The listing builds one solid part. Answer for the finished solid, in the listing's coordinates (mm). A direction names the side the tool comes from. Give positions to 0.01 mm unless a question says otherwise; leave off trailing zeros. Write each loop counter-clockwise with the first axis right and the second up, starting at its lowest first coordinate (ties: lowest second). Pieces come first, ordered by that corner, then holes.
```python
from build123d import *

# Parameters (mm, degrees)
SZKIC1_R                      = 8.5
SZKIC1_R_2                    = 4.2
DODANIE_WYCI_GNI_CIE1_DEPTH   = 30
SZKIC1_W                      = 60
SZKIC1_H                      = 5
DODANIE_WYCI_GNI_CIE1_2_DEPTH = 30
DODANIE_WYCI_GNI_CIE2_DEPTH   = 5
SZKIC3_W                      = 6
SZKIC3_H                      = 22
DODANIE_WYCI_GNI_CIE3_DEPTH   = 26
DODANIE_WYCI_GNI_CIE4_DEPTH   = 5
WYTNIJ_WYCI_GNI_CIE1_REACH    = 62.052
SZKIC5_R                      = 2
WYTNIJ_WYCI_GNI_CIE2_REACH    = 62.052
SZKIC6_W                      = 10.270986067
SZKIC6_H                      = 1.5
SZKIC7_W                      = 9.24961725
SZKIC7_H                      = 2.5
DODANIE_WYCI_GNI_CIE5_DEPTH   = 30
SZKIC8_R                      = 2
WYTNIJ_WYCI_GNI_CIE3_DEPTH    = 30


with BuildPart() as part:
    # Szkic1 → Dodanie-wyci_gni_cie1 (new body)
    with BuildSketch(Plane(origin=(0, 0, 0), x_dir=(1, 0, 0), z_dir=(0, 1, 0))):
        with Locations(Location((0, 34, 0), (0, 0, 270))):
            Circle(SZKIC1_R)
        with Locations(Location((0, 34, 0), (0, 0, 270))):
            Circle(SZKIC1_R_2, mode=Mode.SUBTRACT)
    extrude(amount=DODANIE_WYCI_GNI_CIE1_DEPTH)



with BuildPart() as body_2:
    # Szkic1 → Dodanie-wyci_gni_cie1 2 (new body)
    with BuildSketch(Plane(origin=(0, 0, 0), x_dir=(1, 0, 0), z_dir=(0, 1, 0))):
        with Locations((0, 2.5)):
            Rectangle(SZKIC1_W, SZKIC1_H)
    extrude(amount=DODANIE_WYCI_GNI_CIE1_2_DEPTH)


with BuildPart() as part_1:
    add(part.part)

    add(body_2.part)  # Dodanie-wyci_gni_cie2 merges body 2
    # Szkic2 → Dodanie-wyci_gni_cie2 (add)
    with BuildSketch(Plane.XZ):
        Polygon((30, -5), (8.5, -34), (0, -25.5), (-8.5, -34), (-30, -5), align=None)
    extrude(amount=-DODANIE_WYCI_GNI_CIE2_DEPTH)

    # Szkic3 → Dodanie-wyci_gni_cie3 (add)
    with BuildSketch(Plane(origin=(0, 30, 0), x_dir=(1, 0, 0), z_dir=(0, 1, 0))):
        with Locations((0, 16)):
            Rectangle(SZKIC3_W, SZKIC3_H)
    extrude(amount=-DODANIE_WYCI_GNI_CIE3_DEPTH)

    # Szkic4 → Dodanie-wyci_gni_cie4 (add)
    with BuildSketch(Plane(origin=(0, 30, 0), x_dir=(1, 0, 0), z_dir=(0, 1, 0))):
        Polygon((0, 26.824162036), (8.5, 34), (30, 5), (-30, 5), (-8.5, 34), align=None)
    extrude(amount=-DODANIE_WYCI_GNI_CIE4_DEPTH)

    # Szkic5 → Wytnij-wyci_gni_cie1 (cut, up to next)
    with BuildSketch(Plane.XY, mode=Mode.PRIVATE) as wytnij_wyci_gni_cie1_sk1:
        with Locations((-20, 15)):
            Circle(SZKIC5_R)
    wytnij_wyci_gni_cie1_tool1 = extrude(wytnij_wyci_gni_cie1_sk1.sketch, amount=-WYTNIJ_WYCI_GNI_CIE1_REACH, mode=Mode.PRIVATE) & part_1.part
    # Szkic5 → Wytnij-wyci_gni_cie1 (cut, up to next)
    with BuildSketch(Plane.XY, mode=Mode.PRIVATE) as wytnij_wyci_gni_cie1_sk2:
        with Locations((20, 15)):
            Circle(SZKIC5_R)
    wytnij_wyci_gni_cie1_tool2 = extrude(wytnij_wyci_gni_cie1_sk2.sketch, amount=-WYTNIJ_WYCI_GNI_CIE1_REACH, mode=Mode.PRIVATE) & part_1.part
    add(wytnij_wyci_gni_cie1_tool1.solids().sort_by_distance((-20, 15, 0))[0], mode=Mode.SUBTRACT)
    add(wytnij_wyci_gni_cie1_tool2.solids().sort_by_distance((20, 15, 0))[0], mode=Mode.SUBTRACT)

    # Szkic6 → Wytnij-wyci_gni_cie2 (cut, up to next)
    with BuildSketch(Plane(origin=(0, 30, 0), x_dir=(1, 0, 0), z_dir=(0, 1, 0)), mode=Mode.PRIVATE) as wytnij_wyci_gni_cie2_sk1:
        with Locations((5.135493034, 34)):
            Rectangle(SZKIC6_W, SZKIC6_H)
    wytnij_wyci_gni_cie2_tool1 = extrude(wytnij_wyci_gni_cie2_sk1.sketch, amount=-WYTNIJ_WYCI_GNI_CIE2_REACH, mode=Mode.PRIVATE) & part_1.part
    add(wytnij_wyci_gni_cie2_tool1.solids().sort_by_distance((5.135493, 30, -34))[0], mode=Mode.SUBTRACT)

    # Szkic7 → Dodanie-wyci_gni_cie5 (add)
    with BuildSketch(Plane(origin=(0, 30, 0), x_dir=(1, 0, 0), z_dir=(0, 1, 0))):
        with Locations((10.375191375, 32)):
            Rectangle(SZKIC7_W, SZKIC7_H)
        with Locations((10.375191375, 36)):
            Rectangle(SZKIC7_W, SZKIC7_H)
    extrude(amount=-DODANIE_WYCI_GNI_CIE5_DEPTH)

    # Szkic8 → Wytnij-wyci_gni_cie3 (cut)
    with BuildSketch(Plane(origin=(0, 0, -37.25), x_dir=(-1, 0, 0), z_dir=(0, 0, -1))):
        with Locations((-11.3, 15)):
            Circle(SZKIC8_R)
    extrude(amount=-WYTNIJ_WYCI_GNI_CIE3_DEPTH, mode=Mode.SUBTRACT)


solid = part_1.part
```
Item 1: A cutting plane is placed at B-B, the plane y = 15. Count the separate pieces of the cut face and the enclosed holes in it, plus the area to 3 significant figures.
Conclusion:
separate pieces: 5
enclosed holes: 0
area: 563 mm2
Item 2: A cutting plane is placed at C-C, the plane x = 7. Give the vertices of the cut face in (y, z).
Conclusion:
outline: (0, -38.82) - (30, -38.82) - (30, -34.75) - (0, -34.75) - close; (0, -33.25) - (30, -33.25) - (30, 0) - (0, 0) - close; hole (5, -29.18) - (25, -29.18) - (25, -5) - (5, -5) - close
Item 3: Consider probe 1 along Z at (x, y) = (8, 11.5); probe 2 along Y at (x, z) = (-13, -26); probe 3 along Z at (x, y) = (0, 11.5). Determine where each line is inside the solid, lowest interval first.
Conclusion:
probe 1: z = -37.25 to -34.75, -33.25 to -30.75, -5 to 0
probe 2: y = 0 to 5, 25 to 30
probe 3: z = -42.5 to -38.2, -29.8 to 0
Item 4: Which of the six approach directions +Z, -Z, +X, -X, +Y, -Y give full straight-line access (tool end or side, diameter ignored) to faces 5 (the face through (11.56, 16.983, -36.018)), 6 (the face through (9, 15, -37.25)), 7 (the face through (20.59, 2.46, -17.69))?
Conclusion:
face 5: -Z
face 6: -Z, +X, +Y, -Y
face 7: +X, +Y, -Y
Item 5: A cutting plane is placed at A-A, the plane x = 0. Give the vertices of the cut face in (y, z), plus the area to 3 significant figures.
Conclusion:
outline: (0, -42.5) - (30, -42.5) - (30, -38.2) - (0, -38.2) - close; (0, -29.8) - (30, -29.8) - (30, 0) - (0, 0) - close
area: 1,020 mm2
Item 6: A cutting plane is placed at D-D, the plane z = -27. Give the vertices of the cut face in (x, y).
Conclusion:
outline: (-13.69, 0) - (13.69, 0) - (13.69, 5) - (4.82, 5) - (4.82, 25) - (13.69, 25) - (13.69, 30) - (-13.69, 30) - (-13.69, 25) - (-4.82, 25) - (-4.82, 5) - (-13.69, 5) - close
Item 7: Determine the mould class of faces 1 (the face through (-19.1, 2.5, -19.7)), 2 (the face through (-17, 15, -5)), 3 (the face through (-2.783, 14.79, -42.031)), 4 (the face through (0, 0, -16)) for opening direction Y: pulls with the +Y half, pulls with the -Y half, needs draft (parallel to the pull), parting line crosses it, or undercut.
Conclusion:
face 1: needs draft
face 2: undercut
face 3: undercut
face 4: pulls with the -Y half
Item 8: Each of these flat-tipped pins is pushed along its axis until it touches: P1, Ø12, axis at x = -23.5, y = 18, coming from the -Z side; P2, Ø10, axis at y = 14, z = -27.5, coming from the -X side; P3, Ø6, axis at x = 14, y = 20, coming from the -Z side; P4, Ø7.5, axis at x = 0, z = -34, coming from the -Y side. Where does it stop, or does it pass through?
Conclusion:
P1: stops at z = -5
P2: stops at x = -8.37
P3: stops at z = -37.25
P4: passes through
